```python
from build123d import *

# Parameters (mm, degrees)
SKETCH1_R           = 2.85
BOSS_EXTRUDE1_DEPTH = 3
SKETCH2_R           = 1.5
BOSS_EXTRUDE2_DEPTH = 8
CHAMFER1_SIZE       = 0.3
CUT_EXTRUDE1_DEPTH  = 2


with BuildPart() as part:
    # Sketch1 → Boss-Extrude1 (new body)
    with BuildSketch(Plane.XY):
        Circle(SKETCH1_R)
    extrude(amount=BOSS_EXTRUDE1_DEPTH)

    # Sketch2 → Boss-Extrude2 (add)
    with BuildSketch(Plane(origin=(0, 0, 0), x_dir=(-1, 0, 0), z_dir=(0, 0, -1))):
        Circle(SKETCH2_R)
    extrude(amount=BOSS_EXTRUDE2_DEPTH)

    # Chamfer1
    chamfer1_edges = [part.edges().sort_by_distance(p)[0] for p in [
        (1.5, 0, -8),
    ]]
    chamfer(chamfer1_edges, length=CHAMFER1_SIZE)

    # Sketch3 → Cut-Extrude1 (cut)
    with BuildSketch(Plane.XY.offset(3)):
        Polygon((0, 1.443375673), (-1.25, 0.721687836), (-1.25, -0.721687836), (0, -1.443375673), (1.25, -0.721687836), (1.25, 0.721687836), align=None)
    extrude(amount=-CUT_EXTRUDE1_DEPTH, mode=Mode.SUBTRACT)


solid = part.part
```
Can you work these out from the model? Positions are in its coordinate system, mm. A direction names the side the tool comes from. Round coordinates to 2 decimals unless told otherwise and drop trailing zeros. Loops run counter-clockwise (first coordinate to the right, second up) from the corner with the lowest first, then second, coordinate; pieces in that order, holes last.
Item 1: Suppose I cut it at B-B, the plane z = 0.5. Write out the boundary of the cut face in (x, y), then the cut area to 3 significant figures.
Item 2: Will this pin go through, and if not, where does the flat tip stop? pin 1 Ø1.5 at (x, z) = (1, -6) entering from +Y.
Item 3: Suppose I cut it at A-A, the plane y = 0. Write out the boundary of the cut face in (x, z).
Item 4: Which directions (+Z, -Z, +X, -X, +Y, -Y) give clear straight access to the entire face, cutting with the end or side of a thin tool? Please do faces 1 (the flat face through (1.25, 0, 2)), 2 (the cylindrical face through (1.5, 0.07, -3.8)), 3 (the flat face through (0, 0, -8)).
Item 5: Suppose I cut it at C-C, the plane x = 1.9. Write out the boundary of the cut face in (y, z).
Item 6: If we mould it in two halves opening along Y, with no side actions, what happens to faces 4 (the flat face through (0.63, 1.08, 2.01)), 5 (the cylindrical face through (-2.262, -1.734, 1.479)), 6 (the flat face through (-0.67, -1.23, 3))? For each: +Y half, -Y half, draft (parallel to the pull), parting line (faces both ways), or undercut.
Item 7: Suppose I cut it at D-D, the plane y = -2.1. Write out the boundary of the cut face in (x, z), then the cut area to 3 significant figures.
Item 8: Please list where these lines run through material, in increasing order: L1, parallel to X at y = -0.8, z = 2; L2, parallel to Z at x = -0.5, y = 0.9; L3, parallel to Z at x = -2.5, y = -1.25.
Reported:
1. outline: circle Ø5.7 at (0, 0)
1. area: 25.5 mm2
2. pin 1: stops at y = 1.48
3. outline: (-2.85, 0) - (-1.5, 0) - (-1.5, -7.7) - (-1.2, -8) - (1.2, -8) - (1.5, -7.7) - (1.5, 0) - (2.85, 0) - (2.85, 3) - (1.25, 3) - (1.25, 1) - (-1.25, 1) - (-1.25, 3) - (-2.85, 3) - close
4. face 1: +Z
4. face 2: -Z
4. face 3: -Z, +X, -X, +Y, -Y
5. outline: (-2.12, 0) - (2.12, 0) - (2.12, 3) - (-2.12, 3) - close
6. face 4: undercut
6. face 5: parting line
6. face 6: draft
7. outline: (-1.93, 0) - (1.93, 0) - (1.93, 3) - (-1.93, 3) - close
7. area: 11.6 mm2
8. L1: x = -2.74 to -1.11, 1.11 to 2.74
8. L2: z = -8 to 1
8. L3: z = 0 to 3
